Study the drawing (mm; zero at the part's minimum x, y, z) and answer. A direction names the side the tool comes from. Round coordinates to 2 decimals unless told otherwise and drop trailing zeros. Order: outer loops, then holes, each group sorted by start corner. A loop starts at its lowest first (then second) coordinate and runs counter-clockwise, first axis right, second up. Notation, with made-up numbers: M 52,-7.75 L 89,-7.75 A11 cw 89,7.25 Z; hole C -25.5,81.25 d1. An arc over 180 degrees is marked long. Put each result on its own line as item: value. Start each with the question number.
1. Which of the six approach directions +Z, -Z, +X, -X, +Y, -Y give full straight-line access (tool end or side, diameter ignored) to the marked faces 4, 5 and 6?
2. The part is cut by section C-C (y = 61.25). Give the vertices of the cut face in (x, z), then the cut area to 3 significant figures.
3. Consider line 1 (Y direction, x = 5, z = 3.55); line 2 (Y direction, x = 53.25, z = 3.3); line 3 (Z direction, x = 4, y = 61). Determine where each line is inside the solid, lowest interval first.
4. The part is cut by section D-D (x = 5). Give the vertices of the cut face in (y, z), then the cut area to 3 significant figures.
5. The part is cut by section B-B (x = 36.5). Give the vertices of the cut face in (y, z).
6. The part is cut by section A-A (z = 15). Give the vertices of the cut face in (x, y).
7. Each of these flat-tipped pins is pushed along its axis until it touches: pin 1 Ø7.5 at (y, z) = (61.25, 15) entering from +X; pin 2 Ø11 at (x, z) = (4.5, 17) entering from +Y; pin 3 Ø5 at (x, y) = (5, 17.5) entering from +Z. Where does it stop, or does it pass through?
8. The mould has two halves that part along X. Classify the marked faces 1, 2 and 3: +X half, -X half, draft (parallel to the pull), parting line (faces both ways), or undercut.
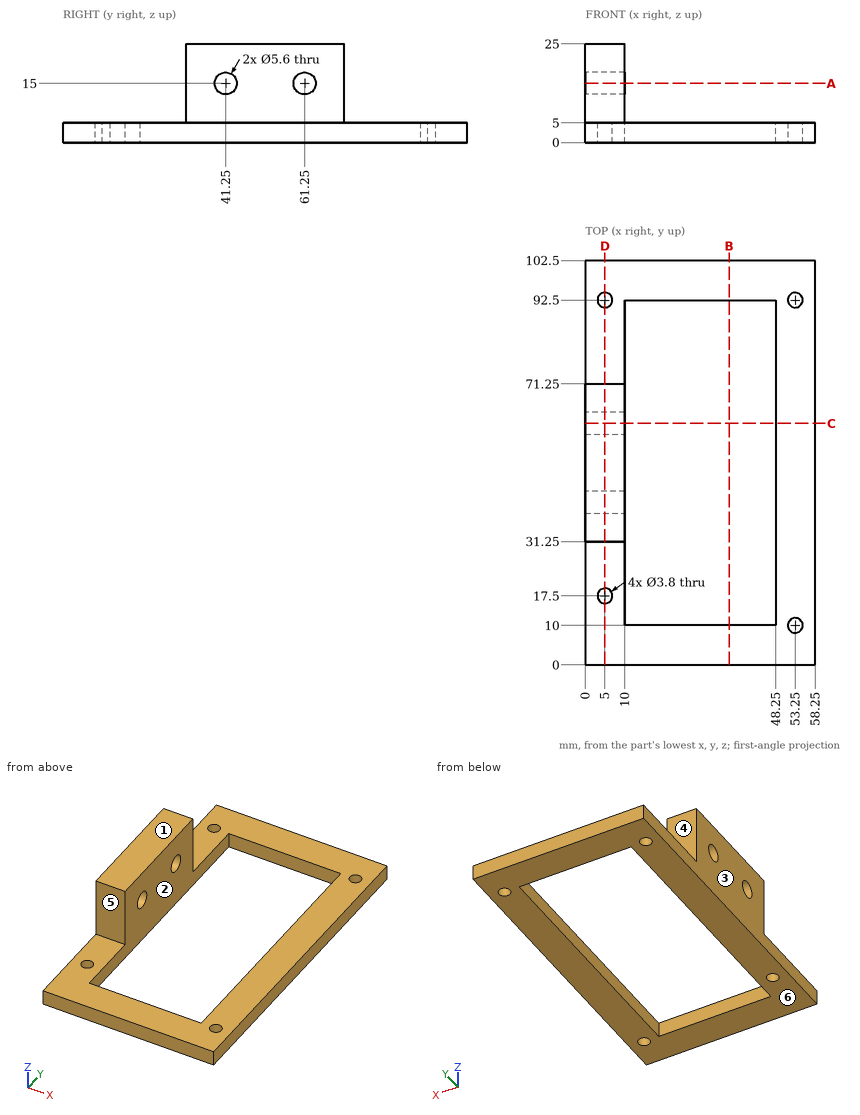
Resolved:
1. face 4: +Z, +X, -X, +Y
1. face 5: +Z, +X, -X, -Y
1. face 6: -Z, +X, -X, +Y, -Y
2. outline: M 0,0 L 10,0 L 10,12.2 L 0,12.2 Z; M 0,17.8 L 10,17.8 L 10,25 L 0,25 Z; M 48.25,0 L 58.25,0 L 58.25,5 L 48.25,5 Z
2. area: 244 mm2
3. line 1: 0 to 15.6, 19.4 to 90.6, 94.4 to 102.5
3. line 2: 0 to 8.1, 11.9 to 90.6, 94.4 to 102.5
3. line 3: 0 to 12.21, 17.79 to 25
4. outline: M 0,0 L 15.6,0 L 15.6,5 L 0,5 Z; M 19.4,0 L 90.6,0 L 90.6,5 L 71.25,5 L 71.25,25 L 31.25,25 L 31.25,5 L 19.4,5 Z; M 94.4,0 L 102.5,0 L 102.5,5 L 94.4,5 Z; hole C 41.25,15 d5.6; hole C 61.25,15 d5.6
4. area: 1,230 mm2
5. outline: M 0,0 L 10,0 L 10,5 L 0,5 Z; M 92.5,0 L 102.5,0 L 102.5,5 L 92.5,5 Z
6. outline: M 0,31.25 L 10,31.25 L 10,38.45 L 0,38.45 Z; M 0,44.05 L 10,44.05 L 10,58.45 L 0,58.45 Z; M 0,64.05 L 10,64.05 L 10,71.25 L 0,71.25 Z
7. pin 1: x = 10
7. pin 2: y = 71.25
7. pin 3: z = 5
8. face 1: draft
8. face 2: undercut
8. face 3: -X half
